Autodesk Inventor part; units mm, degrees
ref_plane "YZ Plane" through (0, 0, 0) normal (1, 0, 0) x (0, 1, 0)
ref_plane "XZ Plane" through (0, 0, 0) normal (0, 1, 0) x (-1, 0, 0)
ref_plane "XY Plane" through (0, 0, 0) normal (0, 0, 1) x (1, 0, 0)
sketch "Sketch1" plane through (0, 0, 0) normal (0, 0, 1) x (1, 0, 0)
  line L0 (0, 0) -> (12.7, 0)
  line L1 (12.7, 0) -> (12.7, 19.05)
  line L2 (12.7, 19.05) -> (0, 19.05)
  line L3 (0, 19.05) -> (0, 0)
  dimension "d0" = 19.05
  dimension "d1" = 12.7
extrude "Extrusion1" add sketch "Sketch1" along normal blind 0.1397
sketch "Sketch2" plane through (0, 0, 0.1397) normal (0, 0, 1) x (1, 0, 0)
  circle A0 centre (6.35, 13.3299) radius 1.905
  line L0 (12.7, 0) -> (12.7, 19.05)
  line L1 (12.7, 19.05) -> (0, 19.05)
  point P0 (0, 0)
  dimension "d4" = 6.35
  dimension "d5" = 5.7201
  dimension "d6" = 3.81
extrude "Extrusion2" cut sketch "Sketch2" against normal blind 0.1397
properties part number "TO220 Thermal Film"
Check sheet for the modelled part. Datum: model origin and axes. Units: mm. Give positions to 0.01 mm unless a question says otherwise; leave off trailing zeros. Order: outer loops, then holes, each group sorted by start corner. A loop starts at its lowest first (then second) coordinate and runs counter-clockwise, first axis right, second up. Notation, with made-up numbers: (-23.5, 14.25) -> (-16.5, 14.25) arc R6 ccw to (-16.5, 20.25) -> close; hole circle Ø5 at (26, 33). An arc over 180 degrees is marked (long way). Use CSV: the item, a comma, the result in double quotes. Start each with the question number.
1) Material ranges on line 1 (Y direction, x = 6.35, z = 0.1); line 2 (Y direction, x = 5, z = 0.1), recorded low to high. Write a range as from..to.
2) Sectioned sample at A-A, the plane x = 6.35. Record the boundary of the cut face in (y, z).
3) Sectioned sample at B-B, the plane z = 0.05. Record the boundary of the cut face in (x, y) (3 decimals).
4) Go/stop test with a flat-tipped pin: P1, Ø6, axis at x = 6.35, y = 13.33, coming from the -Z side. Record where the tip stops, or that it passes through.
Recorded:
1,line 1,"0..11.42, 15.23..19.05"
1,line 2,"0..11.99, 14.67..19.05"
2,outline,"(0, 0) -> (11.42, 0) -> (11.42, 0.14) -> (0, 0.14) -> close; (15.23, 0) -> (19.05, 0) -> (19.05, 0.14) -> (15.23, 0.14) -> close"
3,outline,"(0, 0) -> (12.7, 0) -> (12.7, 19.05) -> (0, 19.05) -> close; hole circle Ø3.81 at (6.35, 13.33)"
4,P1,"z = 0"
